Check sheet for the modelled part. Datum: model origin and axes. Units: mm. A direction names the side the tool comes from. Coordinates: 2 decimals unless noted, no trailing zeros. Loops run counter-clockwise (first coordinate to the right, second up) from the corner with the lowest first, then second, coordinate; pieces in that order, holes last. Notation, with made-up numbers: M 87.5,4.5 L 92.5,4.5 A19 ccw 92.5,16.5 Z; hole C 53,-14.75 d4. An arc over 180 degrees is marked long. Answer in a Markdown table with one row per item. Add a question column.
```python
from build123d import *

# Parameters (mm, degrees)
SKETCH1_W           = 66.04
SKETCH1_H           = 92.964
BOSS_EXTRUDE1_DEPTH = 23.368
SKETCH3_W           = 66.04
SKETCH3_H           = 1.016
BOSS_EXTRUDE2_DEPTH = 17.018


with BuildPart() as part:
    # Sketch1 → Boss-Extrude1 (new body)
    with BuildSketch(Plane.XY):
        Rectangle(SKETCH1_W, SKETCH1_H)
    extrude(amount=BOSS_EXTRUDE1_DEPTH)

    # Sketch3 → Boss-Extrude2 (add)
    with BuildSketch(Plane(origin=(0, 46.482, 0), x_dir=(1, 0, 0), z_dir=(0, 1, 0))):
        with Locations((0, -0.508)):
            Rectangle(SKETCH3_W, SKETCH3_H)
    extrude(amount=BOSS_EXTRUDE2_DEPTH)


solid = part.part
```
Q1. Go/stop test with flat-tipped pins: pin 1 (8 mm diameter, centred on x = -13.5, z = 14.5, fed in from +Y); pin 2 (5 mm diameter, centred on x = 3, y = 55.5, fed in from +Z). Record where each tip stops, or that it passes through.
Q2. Cross-section at B-B (y = 49.5). Record the cut outline in (x, z).
Q3. Thickness scan on L1, parallel to Y at x = -4.5, z = 10; L2, parallel to Z at x = -8.5, y = 48. Record the ranges inside material, lowest first.
Q4. Cross-section at C-C (z = 9). Record the cut outline in (x, y).
Q5. Access from +Z, -Z, +X, -X, +Y, -Y to the whole of each face (thin tool, end or side, straight path). Record for faces 1 (the face through (0, 55, 1.016)), 2 (the face through (-33.02, 8, 12)).
Q6. Cross-section at A-A (x = 13). Record the cut outline in (y, z).
Answer key:
| question | item | result |
|---|---|---|
| 1 | pin 1 | y = 46.48 |
| 1 | pin 2 | z = 1.02 |
| 2 | outline | M -33.02,0 L 33.02,0 L 33.02,1.02 L -33.02,1.02 Z |
| 3 | L1 | -46.48 to 46.48 |
| 3 | L2 | 0 to 1.02 |
| 4 | outline | M -33.02,-46.48 L 33.02,-46.48 L 33.02,46.48 L -33.02,46.48 Z |
| 5 | face 1 | +Z, +X, -X, +Y |
| 5 | face 2 | +Z, -Z, -X, +Y, -Y |
| 6 | outline | M -46.48,0 L 63.5,0 L 63.5,1.02 L 46.48,1.02 L 46.48,23.37 L -46.48,23.37 Z |
